CAD build for the part. Positions are in the model's coordinates, mm. Coordinates: 2 decimals unless noted, no trailing zeros. Loops run counter-clockwise (first coordinate to the right, second up) from the corner with the lowest first, then second, coordinate; pieces in that order, holes last. Notation, with made-up numbers: (-15, 77.25) -> (-3, 77.25) arc R25 ccw to (-3, 111.25) -> close; hole circle Ø9 at (-10, -0.5). An arc over 180 degrees is marked (long way). Answer as CSV lines item,"result". Start each with the question number.
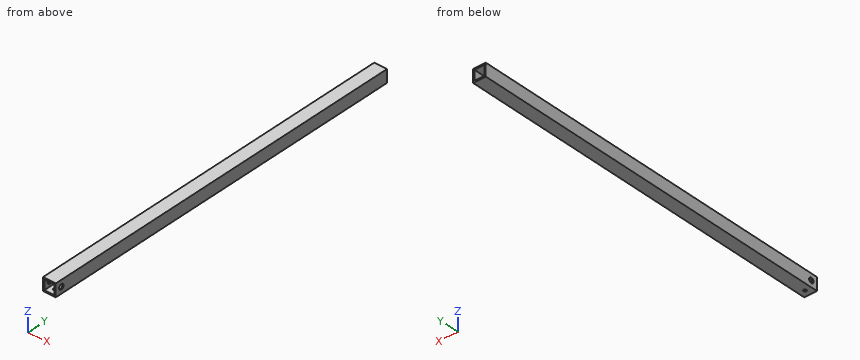
Autodesk Inventor part; units mm, degrees
ref_plane "作業平面1" through (0, 0, 5) normal (1, 0, 0) x (0, 0, -1)
ref_plane "YZ Plane" through (0, 0, 0) normal (1, 0, 0) x (0, 1, 0)
ref_plane "XZ Plane" through (0, 0, 0) normal (0, 1, 0) x (-1, 0, 0)
sketch "スケッチ1" plane through (0, 0, 0) normal (0, 1, 0) x (-1, 0, 0)
  line L0 (5, 5) -> (-5, 5)
  line L1 (-5, 5) -> (-5, -5)
  line L2 (-5, -5) -> (5, -5)
  line L3 (5, -5) -> (5, 5)
  line L4 (4, 4) -> (-4, 4)
  line L5 (-4, 4) -> (-4, -4)
  line L6 (-4, -4) -> (4, -4)
  line L7 (4, -4) -> (4, 4)
  line L8 (5, 5) -> (-5, -5) construction
  line L9 (-5, 5) -> (5, -5) construction
  point P0 (0, 0)
  point P1 (0, 0)
  point P2 (0, 0)
  dimension "d0" = 10
  dimension "d1" = 10
  dimension "d2" = 1
extrude "押し出し1" add sketch "スケッチ1" along normal blind 300
sketch "スケッチ2" plane through (5, 0, 5) normal (1, 0, 0) x (0, 0, -1)
  line L0 (0, 0) -> (10, 0)
  point P0 (5, 0)
  point P1 (5, 10)
  point P2 (5, 0)
  dimension "d5" = 10
hole "穴1" at (5, 10, 0) direction (-1, 0, 0) diameter 4 depth 10
ref_plane "作業平面1" through (0, 0, 5) normal (1, 0, 0) x (0, 0, -1)
sketch "スケッチ3" plane through (-5, 0, -5) normal (-1, 0, 0) x (0, 0, 1)
  line L0 (10, 0) -> (10, 300)
  line L1 (0, 0) -> (10, 0)
  line L2 (10, 0) -> (10, 5)
  line L3 (10, 5) -> (0, 5)
  line L4 (0, 5) -> (0, 0)
  point P0 (5, 0)
  dimension "d13" = 5
extrude "押し出し2" cut sketch "スケッチ3" against normal blind 25.4
sketch "スケッチ5" plane through (5, 300, -5) normal (0, 0, -1) x (-1, 0, 0)
  line L0 (0, -295) -> (0, 0)
  line L1 (0, -295) -> (10, -295)
  point P0 (5, -300)
  point P1 (5, -290)
  dimension "d16" = 5
  dimension "d17" = 5
hole "穴2" at (0, 10, -5) direction (0, 0, 1) diameter 2.459 depth 1
ref_plane "作業平面3" through (-5, 300, 0) normal (0, 0, 1) x (1, 0, 0)
properties part number "stick" material "アルミニウム 6061"
Q1. Saw through at B-B (y = 122). List the corners of the cut face in (x, z), and give its area (3 significant figures).
Q2. Pin check, flat tip, straight feed: pin 1 Ø1.5 at (x, y) = (0, 10) entering from -Z. Stop position of the tip, or through.
Q3. Probe probe 1 along X at (y, z) = (173, 0.5); probe 2 along Y at (x, z) = (-4.2, 0). List the from-to ranges inside material, lowest first. Write a range as from..to.
Q4. Saw through at A-A (z = 0). List the corners of the cut face in (x, y), and give its area (3 significant figures).
Ans:
1,outline,"(-5, -5) -> (5, -5) -> (5, 5) -> (-5, 5) -> close; hole (-4, -4) -> (4, -4) -> (4, 4) -> (-4, 4) -> close"
1,area,"36.0 mm²"
2,pin 1,"stops at z = 4"
3,probe 1,"x = -5..-4, 4..5"
3,probe 2,"y = 5..8, 12..300"
4,outline,"(-5, 5) -> (-4, 5) -> (-4, 8) -> (-5, 8) -> close; (-5, 12) -> (-4, 12) -> (-4, 300) -> (-5, 300) -> close; (4, 5) -> (5, 5) -> (5, 8) -> (4, 8) -> close; (4, 12) -> (5, 12) -> (5, 300) -> (4, 300) -> close"
4,area,"582 mm²"
